Verification items for the finished model (mm, model axes). Face numbers are marked on the shaded views. Give positions to 0.01 mm unless a question says otherwise; leave off trailing zeros. Write each loop counter-clockwise with the first axis right and the second up, starting at its lowest first coordinate (ties: lowest second). Pieces come first, ordered by that corner, then holes. Notation, with made-up numbers: (56.5, -27) -> (85.5, -27) arc R28 ccw to (85.5, 5) -> close; hole circle Ø11 at (-28.75, 81). An arc over 180 degrees is marked (long way). Use one line per item in the form item = value. Start each with the question number.
(1) Section check C-C, the plane x = 20. Record the cut outline in (y, z), plus the area to 3 significant figures.
(2) Section check B-B, the plane y = -58. Record the cut outline in (x, z), plus the area to 3 significant figures.
(3) Scan lines: L1, parallel to X at y = -69.5, z = -8.5; L2, parallel to Z at x = 10, y = -60.5; L3, parallel to Z at x = 4, y = -212.5. Record each from-to range of solid material in increasing order.
(4) Depth check by flat-ended pin: pin 1 Ø3 at (x, y) = (18, -269.5) entering from +Z; pin 2 Ø2 at (y, z) = (-267, -5) entering from +X; pin 3 Ø5.5 at (y, z) = (-88.5, -8) entering from -X. Enter the tip coordinate at first touch or a pass-through.
(5) Release check for a two-part mould opening along X. For the marked faces 1 and 2 record: pulls with the +X half, pulls with the -X half, needs draft (parallel to the pull), parting line crosses it, or undercut.
(6) Section check A-A, the plane z = -4. Record the cut outline in (x, y), plus the area to 3 significant figures.
from build123d import *

# Parameters (mm, degrees)
F1_DEPTH = 300


with BuildPart() as f1:
    # F0 (on Front) → F1 (new body)
    with BuildSketch(Plane.XZ):
        with BuildLine():
            Line((4.5, 0), (0, 0))
            Line((0, 0), (0, -1))
            Line((0, -1), (4.5, -1))
            Line((4.5, -1), (4.5, -12))
            ThreePointArc((4.5, -12), (5.085786, -13.414214), (6.5, -14))
            Line((6.5, -14), (28.5, -14))
            ThreePointArc((28.5, -14), (29.914214, -13.414214), (30.5, -12))
            Line((30.5, -12), (30.5, -1))
            Line((30.5, -1), (35, -1))
            Line((35, -1), (35, 0))
            Line((35, 0), (30.5, 0))
            ThreePointArc((30.5, 0), (29.792893, -0.292893), (29.5, -1))
            Line((29.5, -1), (29.5, -12))
            ThreePointArc((29.5, -12), (29.207107, -12.707107), (28.5, -13))
            Line((28.5, -13), (6.5, -13))
            ThreePointArc((6.5, -13), (5.792893, -12.707107), (5.5, -12))
            Line((5.5, -12), (5.5, -1))
            ThreePointArc((5.5, -1), (5.207107, -0.292893), (4.5, 0))
        make_face()
    extrude(amount=F1_DEPTH)


solid = f1.part
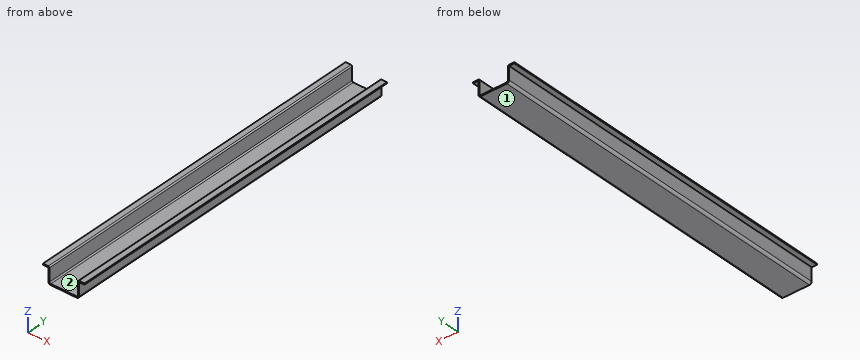
Completed:
q1.outline = (-300, -14) -> (0, -14) -> (0, -13) -> (-300, -13) -> close
q1.area = 300 mm²
q2.outline = (0, -1) -> (4.5, -1) -> (4.5, -12) arc R2 ccw to (6.5, -14) -> (28.5, -14) arc R2 ccw to (30.5, -12) -> (30.5, -1) -> (35, -1) -> (35, 0) -> (30.5, 0) arc R1 ccw to (29.5, -1) -> (29.5, -12) arc R1 cw to (28.5, -13) -> (6.5, -13) arc R1 cw to (5.5, -12) -> (5.5, -1) arc R1 ccw to (4.5, 0) -> (0, 0) -> close
q2.area = 59.3 mm²
q3.L1 = 4.5 to 5.5, 29.5 to 30.5
q3.L2 = -14 to -13
q3.L3 = -1 to 0
q4.pin_1 = -13
q4.pin_2 = 30.5
q4.pin_3 = 4.5
q5.face_1 = needs draft
q5.face_2 = undercut
q6.outline = (4.5, -300) -> (5.5, -300) -> (5.5, 0) -> (4.5, 0) -> close; (29.5, -300) -> (30.5, -300) -> (30.5, 0) -> (29.5, 0) -> close
q6.area = 600 mm²
